The figure shows three views and two pictorial views of one solid part (mm, origin at its lowest corner). Answer the questions. A direction names the side the tool comes from. Round coordinates to 2 decimals unless told otherwise and drop trailing zeros. Write each loop counter-clockwise with the first axis right and the second up, starting at its lowest first coordinate (ties: lowest second). Pieces come first, ordered by that corner, then holes. Notation, with made-up numbers: (57, -37) -> (67, -37) arc R24 cw to (67, -17) -> close; hole circle Ø9 at (79.5, -17). An arc over 180 degrees is marked (long way). One line per item, written item: value.
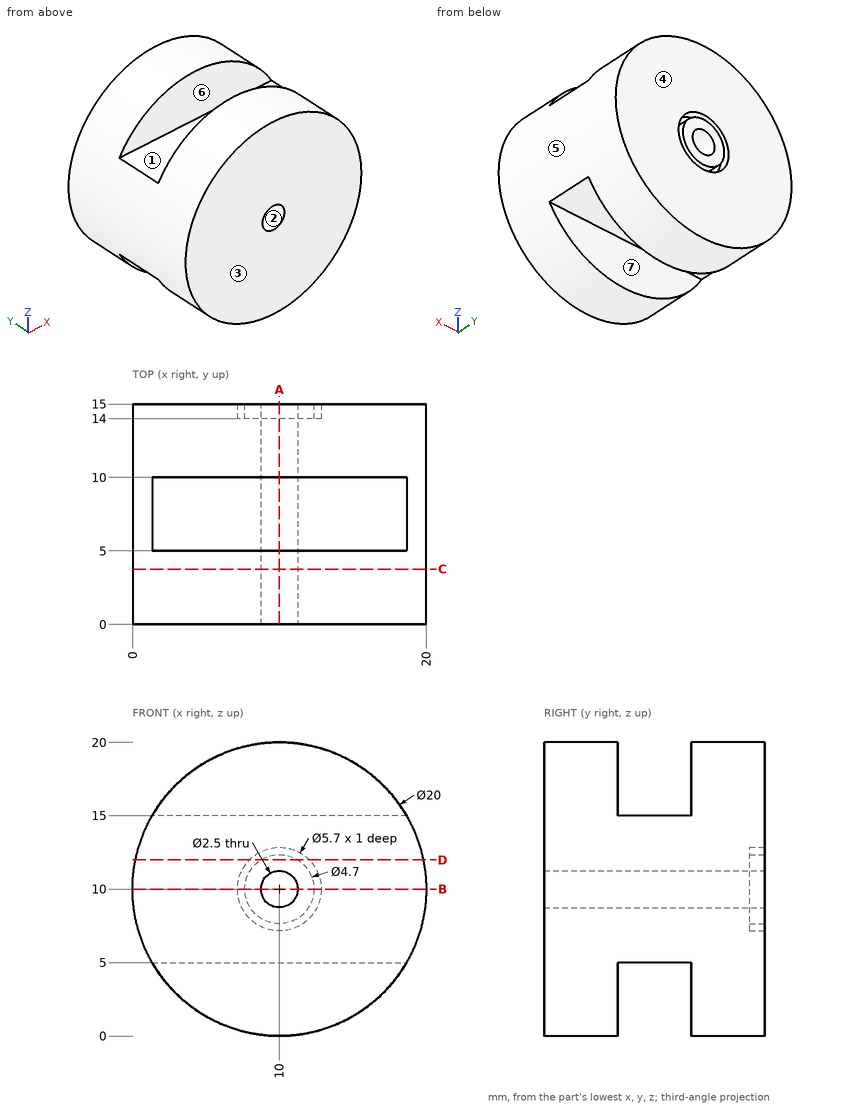
(1) Consider probe 1 along Z at (x, y) = (10, 14.8); probe 2 along Y at (x, z) = (5.25, 4.25). Determine where each line is inside the solid, lowest interval first.
Reported:
probe 1: z = 0 to 7.15, 7.65 to 8.75, 11.25 to 12.35, 12.85 to 20
probe 2: y = 0 to 5, 10 to 15
(2) Find section C-C on y = 3.75. Give the vertices of the cut face in (x, z).
Reported:
outline: circle Ø20 at (10, 10); hole circle Ø2.5 at (10, 10)
(3) Flat-ended cylindrical pins translate along their axes: pin 1 Ø10 at (x, z) = (3.5, 13) entering from -Y; pin 2 Ø3 at (y, z) = (9.5, 15) entering from +X; pin 3 Ø2.5 at (x, y) = (9.5, 6.5) entering from +Z; pin 4 Ø5 at (y, z) = (9.5, 5.5) entering from -X. Find the tip coordinate at first contact, or state that the pin passes through.
Reported:
pin 1: stops at y = 0
pin 2: stops at x = 19.37
pin 3: stops at z = 15
pin 4: stops at x = 0.2
(4) Find section B-B on z = 10. Give the vertices of the cut face in (x, y), plus the area to 4 significant figures.
Reported:
outline: (0, 0) -> (8.75, 0) -> (8.75, 15) -> (7.65, 15) -> (7.65, 14) -> (7.15, 14) -> (7.15, 15) -> (0, 15) -> close; (11.25, 0) -> (20, 0) -> (20, 15) -> (12.85, 15) -> (12.85, 14) -> (12.35, 14) -> (12.35, 15) -> (11.25, 15) -> close
area: 261.5 mm2
(5) Find section A-A on x = 10. Give the vertices of the cut face in (y, z).
Reported:
outline: (0, 0) -> (5, 0) -> (5, 5) -> (10, 5) -> (10, 0) -> (15, 0) -> (15, 7.15) -> (14, 7.15) -> (14, 7.65) -> (15, 7.65) -> (15, 8.75) -> (0, 8.75) -> close; (0, 11.25) -> (15, 11.25) -> (15, 12.35) -> (14, 12.35) -> (14, 12.85) -> (15, 12.85) -> (15, 20) -> (10, 20) -> (10, 15) -> (5, 15) -> (5, 20) -> (0, 20) -> close
(6) For a pull along Y with two mould halves and no side action, classify the marked faces 1, 2, 3 and 4 as pulls with the +Y half, pulls with the -Y half, needs draft (parallel to the pull), parting line crosses it, or undercut.
Reported:
face 1: undercut
face 2: needs draft
face 3: pulls with the -Y half
face 4: pulls with the +Y half
(7) A tool of negligible diameter and unlimited length cuts with its end or side. For the marked faces 5, 6 and 7, from which of +Z, -Z, +X, -X, +Y, -Y can it reach the whole face along a straight path? Write none if from no direction.
Reported:
face 5: +Y, -Y
face 6: +Z, +X, -X
face 7: -Z, +X, -X
(8) Find section D-D on z = 12. Give the vertices of the cut face in (x, y), plus the area to 3 significant figures.
Reported:
outline: (0.2, 0) -> (19.8, 0) -> (19.8, 15) -> (12.03, 15) -> (12.03, 14) -> (11.23, 14) -> (11.23, 15) -> (8.77, 15) -> (8.77, 14) -> (7.97, 14) -> (7.97, 15) -> (0.2, 15) -> close
area: 292 mm2
